Can you work these out from the model? Positions are in its coordinate system, mm. A direction names the side the tool comes from. Give positions to 0.01 mm unless a question says otherwise; leave off trailing zeros. Loops run counter-clockwise (first coordinate to the right, second up) from the corner with the lowest first, then second, coordinate; pieces in that order, holes last. Notation, with made-up numbers: M 70.5,36.5 L 103.5,36.5 A13 ccw 103.5,40.5 Z; hole C 45.5,-6.75 d2. An arc over 180 degrees is marked long. Put each result on its own line as item: value. Start each with the question number.
1) Imagine slicing it at B-B (x = 456). Write out the boundary of the cut face in (y, z), then the cut area to 3 significant figures.
2) Imagine slicing it at C-C (y = 163). Write out the boundary of the cut face in (x, z).
3) Imagine slicing it at A-A (z = 4.5). State how many separate pieces and enclosed holes the cut face has, then the cut area to 3 significant figures.
4) For P1, Ø1.5, axis at y = 328, z = 14, coming from the +X side; P2, Ø6, axis at y = 327, z = 5, coming from the -X side; P3, Ø1.5, axis at y = 359, z = 7.5, coming from the -X side, each with a flat end and sliding along its axis, tell me the tip position at first contact or that it passes through.
5) If we mould it in two halves opening along Y, with no side actions, what happens to faces 4 (the flat face through (195.732, 356.958, 8.874)), 5 (the flat face through (758, 280, 18)), 6 (the flat face through (1396.582, 405.334, 8.874)), 7 (the flat face through (64.5, 278.31, 8.87))? For each: +Y half, -Y half, draft (parallel to the pull), parting line (faces both ways), or undercut.
6) For faces 1 (the flat face through (1462.846, 278.949, 8.874)), 2 (the flat face through (1297.07, 507.12, 8.87)), 3 (the flat face through (1412.673, 415.58, 8.874)), which set-ups out of +Z, -Z, +X, -X, +Y, -Y let a thin tool reach every point of the face, with its end or its side?
7) Please list where these lines run through material, in increasing order: line 1 along X through (y, z) = (471.5, 2.75); line 2 along X through (y, z) = (441.5, 15); line 3 along X through (y, z) = (241.5, 10). Write a range as from..to.
Autodesk Inventor part; units mm, degrees
ref_plane "YZ Plane" through (0, 0, 0) normal (1, 0, 0) x (0, 1, 0)
ref_plane "XZ Plane" through (0, 0, 0) normal (0, 1, 0) x (-1, 0, 0)
ref_plane "XY Plane" through (0, 0, 0) normal (0, 0, 1) x (1, 0, 0)
sketch "CONTOURS" plane through (0, 0, 0) normal (0, 0, 1) x (1, 0, 0)
  arc A0 (122.9585, 280.6191) -> (147.7621, 282.3295) centre (134.7234, 290.7105) ccw
  line L0 (147.7621, 282.3295) -> (245.0646, 433.7067)
  arc A1 (245.0646, 433.7067) -> (237.169, 456.7096) centre (232.0259, 442.0877) ccw
  line L1 (237.169, 456.7096) -> (221.2353, 462.314)
  arc A2 (214.3157, 484.5154) -> (221.2353, 462.314) centre (226.0465, 475.9926) ccw
  line L2 (214.3157, 484.5154) -> (246.7015, 529.0906)
  arc A3 (246.7015, 529.0906) -> (1281.107, 529.0906) centre (763.9042, 1241.8098) ccw
  line L3 (1281.107, 529.0906) -> (1313.4927, 484.5154)
  arc A4 (1313.4927, 484.5154) -> (1338.3495, 484.2164) centre (1326.0325, 493.6261) ccw
  line L4 (1338.3495, 484.2164) -> (1348.6034, 497.6384)
  arc A5 (1371.3515, 498.0135) -> (1348.6034, 497.6384) centre (1360.1257, 488.8357) ccw
  line L5 (1371.3515, 498.0135) -> (1485.2517, 358.6952)
  arc A6 (1479.6031, 336.133) -> (1485.2517, 358.6952) centre (1474.0258, 349.5174) ccw
  line L6 (1479.6031, 336.133) -> (1452.9579, 325.03)
  arc A7 (1452.9579, 325.03) -> (1446.3801, 301.6117) centre (1458.9198, 310.7224) ccw
  line L7 (1446.3801, 301.6117) -> (1479.7785, 255.6428)
  arc A8 (48.0301, 255.6429) -> (1479.7785, 255.6428) centre (763.9044, 1242.1407) ccw
  line L8 (48.0301, 255.6429) -> (81.4284, 301.6117)
  arc A9 (104.1651, 302.5292) -> (81.4284, 301.6117) centre (93.1592, 293.0889) ccw
  line L9 (104.1651, 302.5292) -> (122.9585, 280.6191)
sketch "HOLES" plane through (0, 0, 0) normal (0, 0, 1) x (1, 0, 0)
  arc A0 (123.1485, 251.2322) -> (122.1121, 256.7934) centre (119.8497, 253.4946) ccw
  line L0 (122.1121, 256.7934) -> (92.4235, 277.1548)
  arc A1 (92.4235, 277.1548) -> (86.8624, 276.1184) centre (90.1611, 273.856) ccw
  line L1 (86.8624, 276.1184) -> (80.6409, 267.0469)
  arc A2 (80.6409, 267.0469) -> (81.6772, 261.4858) centre (83.9396, 264.7845) ccw
  line L2 (116.9269, 242.1607) -> (123.1485, 251.2322)
  arc A3 (111.3658, 241.1244) -> (116.9269, 242.1607) centre (113.6282, 244.4231) ccw
  line L3 (264.0494, 464.2922) -> (234.3609, 484.6537)
  arc A4 (233.3245, 490.2148) -> (234.3609, 484.6537) centre (236.6232, 487.9524) ccw
  line L4 (233.3245, 490.2148) -> (239.546, 499.2863)
  arc A5 (245.1072, 500.3226) -> (239.546, 499.2863) centre (242.8448, 497.0239) ccw
  line L5 (245.1072, 500.3226) -> (274.7957, 479.9612)
  arc A6 (275.8321, 474.4001) -> (274.7957, 479.9612) centre (272.5334, 476.6625) ccw
  line L6 (275.8321, 474.4001) -> (269.6106, 465.3286)
  arc A7 (264.0494, 464.2922) -> (269.6106, 465.3286) centre (266.3118, 467.591) ccw
  line L7 (1443.1181, 358.0576) -> (1448.6625, 362.3307)
  arc A8 (1448.6625, 362.3307) -> (1449.389, 367.9407) centre (1446.2207, 365.4989) ccw
  line L8 (1449.389, 367.9407) -> (1374.9151, 464.5722)
  arc A9 (1374.9151, 464.5722) -> (1369.3051, 465.2986) centre (1371.7469, 462.1304) ccw
  line L9 (1369.3051, 465.2986) -> (1360.5924, 458.5838)
  arc A10 (1360.5924, 458.5838) -> (1359.866, 452.9738) centre (1363.0342, 455.4155) ccw
  line L10 (1359.866, 452.9738) -> (1434.3398, 356.3423)
  arc A11 (1434.3398, 356.3423) -> (1439.9498, 355.6158) centre (1437.5081, 358.7841) ccw
  line L11 (1439.9498, 355.6158) -> (1443.1181, 358.0576)
  line L12 (81.6772, 261.4858) -> (111.3658, 241.1244)
sketch "LETTERS" plane through (0, 0, 0) normal (0, 0, 1) x (1, 0, 0)
  line L0 (274.8207, 322.605) -> (262.022, 329.8103)
  line L1 (262.022, 329.8103) -> (252.3047, 312.5498)
  line L2 (252.3047, 312.5498) -> (265.1034, 305.3445)
extrude "Extrusion1" add sketch "CONTOURS" along normal blind 18
extrude "Extrusion2" cut sketch "HOLES" along normal blind 18
properties part number "Platform E2" material "Wood (Birch)"
Recorded:
1. outline: M 62.8,0 L 416.79,0 L 416.79,18 L 62.8,18 Z
1. area: 6,370 mm²
2. outline: M 197.24,0 L 1330.57,0 L 1330.57,18 L 197.24,18 Z
3. separate pieces: 1
3. enclosed holes: 3
3. area: 441,000 mm²
4. P1: x = 1461.89
4. P2: x = 174.55
4. P3: x = 196.56
5. face 4: undercut
5. face 5: draft
5. face 6: undercut
5. face 7: +Y half
6. face 1: +Z, -Z, +X
6. face 2: +Z, -Z, +Y
6. face 3: +Z, -Z
7. line 1: 212.26..253.54, 273.84..337.18, 1190.62..1393.03
7. line 2: 247.51..396.52, 1131.29..1368.71, 1392.7..1417.55
7. line 3: 67.94..110.82, 116.36..1459.87
